The figure shows three views and two pictorial views of one solid part (mm, origin at its lowest corner). Answer the questions. A direction names the side the tool comes from. Coordinates: 2 decimals unless noted, no trailing zeros. Order: outer loops, then holes, each group sorted by start corner. A loop starts at its lowest first (then second) coordinate and runs counter-clockwise, first axis right, second up. Notation, with made-up numbers: M 59,-30 L 84,-30 A21 ccw 84,6 Z; hole C 64,85.5 d7. An arc over 180 degrees is marked long. Use a Markdown table: item, result.
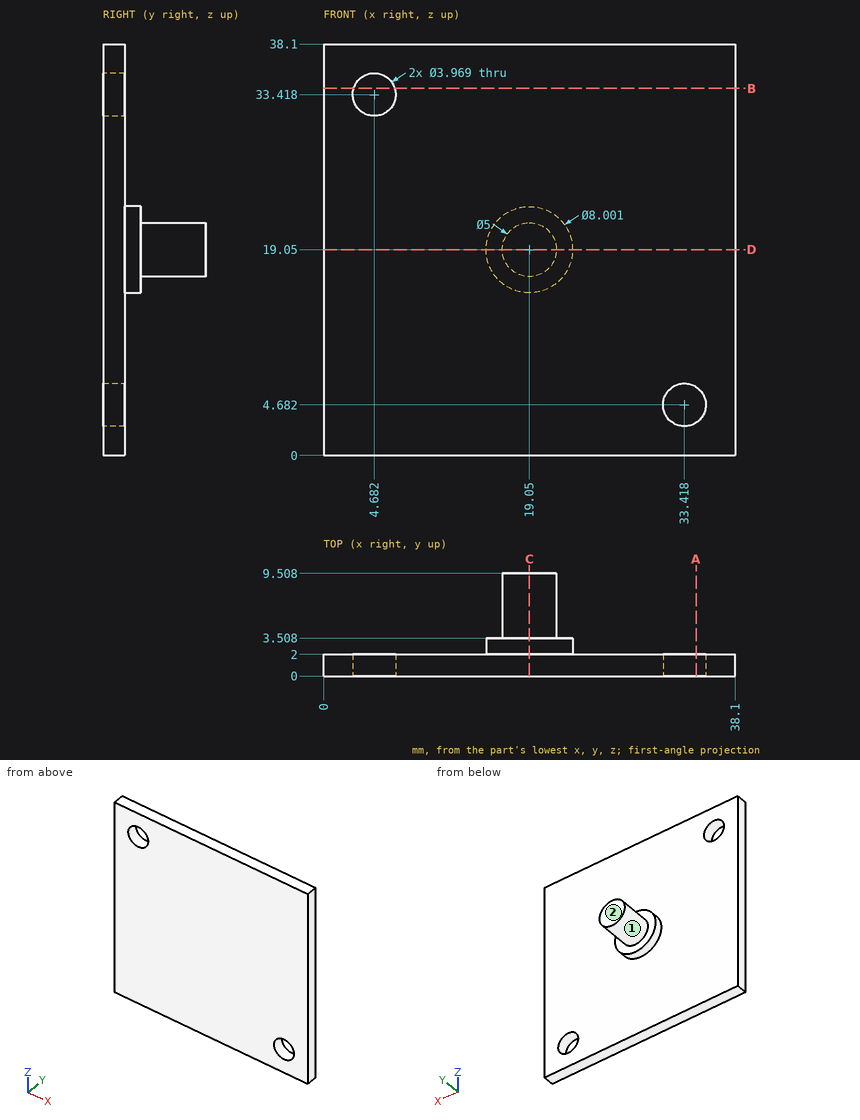
1. Section C-C on x = 19.05 is taken. Determine the outline of the cut face in (y, z), then the cut area to 3 significant figures.
Answers below:
| item | result |
|---|---|
| outline | M 0,0 L 2,0 L 2,15.05 L 3.51,15.05 L 3.51,16.55 L 9.51,16.55 L 9.51,21.55 L 3.51,21.55 L 3.51,23.05 L 2,23.05 L 2,38.1 L 0,38.1 Z |
| area | 118 mm² |
2. Flat-ended cylindrical pins translate along their axes: P1, Ø4.5, axis at x = 4.68, z = 33.42, coming from the +Y side; P2, Ø5, axis at x = 22.5, y = 6.5, coming from the +Z side. Find the tip coordinate at first contact, or state that the pin passes through.
Answers below:
| item | result |
|---|---|
| P1 | y = 2 |
| P2 | z = 21.36 |
3. For the marked faces 1 and 2, determine the directions among +Z, -Z, +X, -X, +Y, -Y from which every point of the face is accessible in a straight line to the end or side of a thin tool.
Answers below:
| item | result |
|---|---|
| face 1 | +Y |
| face 2 | +Z, -Z, +X, -X, +Y |
4. Section B-B on z = 34 is taken. Determine the outline of the cut face in (x, y) (1 decimal).
Answers below:
| item | result |
|---|---|
| outline | M 0,0 L 2.8,0 L 2.8,2 L 0,2 Z; M 6.6,0 L 38.1,0 L 38.1,2 L 6.6,2 Z |
5. Section A-A on x = 34.5 is taken. Determine the outline of the cut face in (y, z) (1 decimal).
Answers below:
| item | result |
|---|---|
| outline | M 0,0 L 2,0 L 2,3 L 0,3 Z; M 0,6.3 L 2,6.3 L 2,38.1 L 0,38.1 Z |
6. Section D-D on z = 19.05 is taken. Determine the outline of the cut face in (x, y), then the cut area to 3 significant figures.
Answers below:
| item | result |
|---|---|
| outline | M 0,0 L 38.1,0 L 38.1,2 L 23.05,2 L 23.05,3.51 L 21.55,3.51 L 21.55,9.51 L 16.55,9.51 L 16.55,3.51 L 15.05,3.51 L 15.05,2 L 0,2 Z |
| area | 118 mm² |
7. Find the intervals of material crossed by probe 1 along Y at (x, z) = (9, 3.5); probe 2 along Z at (x, y) = (22, 2.25), in increasing order.
Answers below:
| item | result |
|---|---|
| probe 1 | 0 to 2 |
| probe 2 | 16.35 to 21.75 |
